Verification items for the finished model (mm, model axes). Face numbers are marked on the shaded views. A direction names the side the tool comes from. Give positions to 0.01 mm unless a question says otherwise; leave off trailing zeros. Order: outer loops, then holes, each group sorted by start corner. A loop starts at its lowest first (then second) coordinate and runs counter-clockwise, first axis right, second up. Notation, with made-up numbers: (62, -10) -> (110, -10) arc R15 ccw to (110, -1) -> close; hole circle Ø8 at (-37.75, 30). An arc over 180 degrees is marked (long way). Return JSON: item names as keys, results as strings. Group by question number.
(1) Tool access check on the marked faces 1 and 2. Record the directions out of +Z, -Z, +X, -X, +Y, -Y that give a thin tool (end or side, any length) a straight path to the whole face; none if there is none.
(2) Cross-section at A-A on x = 562. Enter the section's corners in (y, z), then the cut area to 3 significant figures.
(3) Cross-section at C-C on y = -238. Enter the section's corners in (x, z).
(4) Cross-section at B-B on z = 782. Enter the section's corners in (x, y).
(5) Thickness scan on line 1 along Z through (x, y) = (1073, -751.5); line 2 along Z through (x, y) = (1159, -297.5). Record the ranges inside material, lowest first.
(6) Depth check by flat-ended pin: pin 1 Ø6 at (y, z) = (-980, 1098) entering from +X; pin 2 Ø4 at (x, y) = (759, -1092) entering from +Z; pin 3 Ø8 at (y, z) = (-494.5, 1018) entering from +X. Enter the tip coordinate at first touch or a pass-through.
from build123d import *

# Parameters (mm, degrees)
F1_DEPTH = 1270
F3_DEPTH = 508


with BuildPart() as f1:
    # F0 (on Front) → F1 (new body)
    with BuildSketch(Plane.XZ):
        Polygon((0, 1524), (0, 0), (1270, 0), (1270, 508), (508, 508), (508, 1524), align=None)
    extrude(amount=F1_DEPTH)

    # F2 (on face) → F3 (join)
    with BuildSketch(Plane(origin=(0, 0, 0), x_dir=(-1, 0, 0), z_dir=(0, 1, 0))):
        Polygon((-508, 508), (-508, 1524), (-1270, 508), align=None)
    extrude(amount=-F3_DEPTH)


solid = f1.part
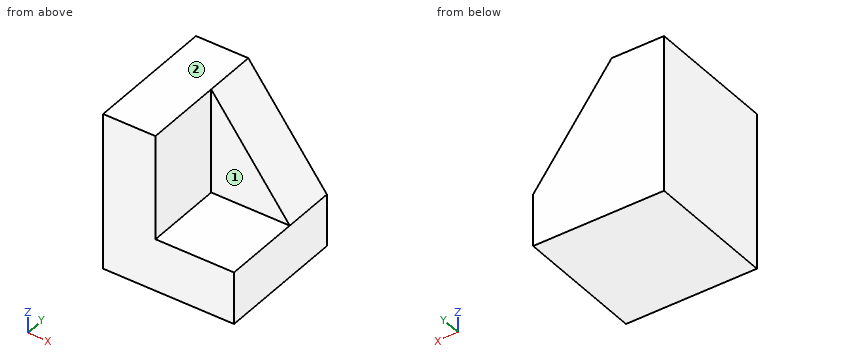
Verdict:
{
 "1": {"face 1": "+Z, +X, -Y", "face 2": "+Z, +X, -X, +Y, -Y"},
 "2": {"outline": "(-1270, 0) -> (0, 0) -> (0, 1452) -> (-508, 1452) -> (-508, 508) -> (-1270, 508) -> close", "area": "1,120,000 mm²"},
 "3": {"outline": "(0, 0) -> (1270, 0) -> (1270, 508) -> (508, 1524) -> (0, 1524) -> close"},
 "4": {"outline": "(0, -1270) -> (508, -1270) -> (508, -508) -> (1064.5, -508) -> (1064.5, 0) -> (0, 0) -> close"},
 "5": {"line 1": "0 to 508", "line 2": "0 to 656"},
 "6": {"pin 1": "x = 508", "pin 2": "z = 508", "pin 3": "x = 890.5"}
}
